from build123d import *

# Parameters (mm, degrees)
SKETCH1_R           = 25
BOSS_EXTRUDE1_DEPTH = 15
CUT_EXTRUDE2_REACH  = 40.406
CUT_EXTRUDE3_DEPTH  = 5


with BuildPart() as part:
    # Sketch1 → Boss-Extrude1 (new body)
    with BuildSketch(Plane(origin=(0, 0, 0), x_dir=(1, 0, 0), z_dir=(0, 1, 0))):
        with Locations(Location((0, 0, 0), (0, 0, 270))):
            Circle(SKETCH1_R)
    extrude(amount=BOSS_EXTRUDE1_DEPTH)

    # Sketch7 → Cut-Extrude2 (cut, up to next)
    with BuildSketch(Plane(origin=(0, 15, 0), x_dir=(1, 0, 0), z_dir=(0, 1, 0)), mode=Mode.PRIVATE) as cut_extrude2_sk1:
        Polygon((0, 5.132643893), (-4.445, 2.566321947), (-4.445, -2.566321947), (0, -5.132643893), (4.445, -2.566321947), (4.445, 2.566321947), align=None)
    cut_extrude2_tool1 = extrude(cut_extrude2_sk1.sketch, amount=-CUT_EXTRUDE2_REACH, mode=Mode.PRIVATE) & part.part
    add(cut_extrude2_tool1.solids().sort_by_distance((0, 15, 0))[0], mode=Mode.SUBTRACT)

    # Sketch8 → Cut-Extrude3 (cut)
    with BuildSketch(Plane.XZ):
        with BuildLine():
            ThreePointArc((2.867832451, 6.276606431), (5.55485913, 5.311303559), (8.103473198, 4.024257195))
            ThreePointArc((8.103473198, 4.024257195), (12.790122891, 3.37163327), (17.445502266, 2.524257195))
            ThreePointArc((17.445502266, 2.524257195), (19.894779582, 1.820498395), (21, -0.475742805))
            ThreePointArc((21, -0.475742805), (19.894779582, -2.771984005), (17.445502266, -3.475742805))
            ThreePointArc((17.445502266, -3.475742805), (12.790122891, -4.32311888), (8.103473198, -4.975742805))
            ThreePointArc((8.103473198, -4.975742805), (5.55485913, -6.262789168), (2.867832451, -7.22809204))
            ThreePointArc((2.867832451, -7.22809204), (0, -7.852228414), (-2.867832451, -7.22809204))
            ThreePointArc((-2.867832451, -7.22809204), (-5.55485913, -6.262789168), (-8.103473198, -4.975742805))
            ThreePointArc((-8.103473198, -4.975742805), (-12.790122891, -4.32311888), (-17.445502266, -3.475742805))
            ThreePointArc((-17.445502266, -3.475742805), (-19.894779582, -2.771984005), (-21, -0.475742805))
            ThreePointArc((-21, -0.475742805), (-19.894779582, 1.820498395), (-17.445502266, 2.524257195))
            ThreePointArc((-17.445502266, 2.524257195), (-12.790122891, 3.37163327), (-8.103473198, 4.024257195))
            ThreePointArc((-8.103473198, 4.024257195), (-5.55485913, 5.311303559), (-2.867832451, 6.276606431))
            ThreePointArc((-2.867832451, 6.276606431), (0, 6.900742805), (2.867832451, 6.276606431))
        make_face()
    extrude(amount=-CUT_EXTRUDE3_DEPTH, mode=Mode.SUBTRACT)


solid = part.part
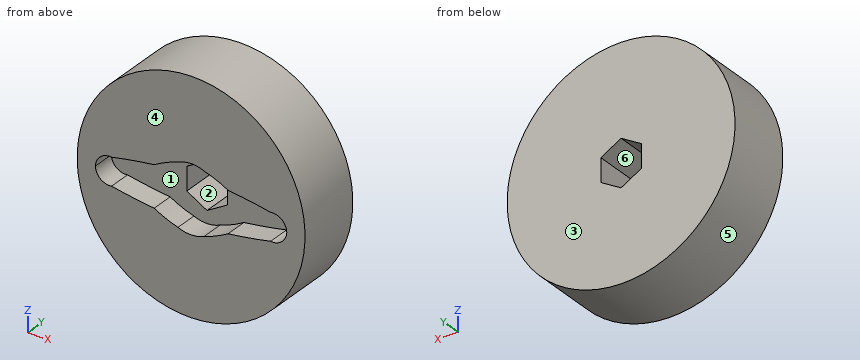
Input: part model. Units: mm. Frame: model coordinates. Face numbers are marked on the shaded views. A direction names the side the tool comes from. Give positions to 0.01 mm unless a question says otherwise; leave off trailing zeros. Loops run counter-clockwise (first coordinate to the right, second up) from the corner with the lowest first, then second, coordinate; pieces in that order, holes last. Notation, with made-up numbers: (14.25, 3) - (52.25, 3) arc R18 ccw to (52.25, 18) - close; hole circle Ø8 at (32, -32.5). An arc over 180 degrees is marked (long way). Use CSV: the item, a comma, the result in double quotes. Start each with the question number.
Item 1: Contact query for flat-ended pins moving along their axis: P1, Ø5, axis at y = 4, z = 5.5, coming from the -X side; P2, Ø1, axis at x = 16, y = 3.5, coming from the +Z side; P3, Ø2.5, axis at y = 8.5, z = 0, coming from the +X side. Output: stop coordinate, or through.
Item 2: Section B-B on z = -6. Return loops of the section in (x, y).
Item 3: Section A-A on y = 2.75. Return loops of the section in (x, z), then the cut area to 3 significant figures.
Item 4: Section D-D on x = -7. Return loops of the section in (y, z), then the cut area to 3 significant figures.
Item 5: Line query: line 1 (X direction, y = 13.5, z = 0) (3 decimals); line 2 (Z direction, x = -3, y = 12); line 3 (Y direction, x = 20, z = 1.5). Output: solid intervals per line, ascending.
Item 6: Mould query, pull axis X, two halves, no side actions, for the marked faces 4, 5 and 6. Classes: pulls with the +X half, pulls with the -X half, needs draft (parallel to the pull), parting line crosses it, or undercut.
Item 7: Reachability of the marked faces 1, 2 and 3 from +Z, -Z, +X, -X, +Y, -Y: full face, straight path, thin tool, end or side. Return the list, or none.
Item 8: Section C-C on y = 7.5. Return loops of the section in (x, z) (3 decimals), then the cut area to 3 significant figures.
Ans:
1,P1,"stops at x = -24.82"
1,P2,"stops at z = 19.62"
1,P3,"stops at x = 25"
2,outline,"(-24.27, 0) - (-6.14, 0) - (-6.14, 5) - (6.14, 5) - (6.14, 0) - (24.27, 0) - (24.27, 15) - (-24.27, 15) - close"
3,outline,"circle Ø50 at (0, 0); hole (-21, -0.48) arc R3.12 ccw to (-17.45, -3.48) arc R113.52 ccw to (-8.1, -4.98) arc R23.27 ccw to (-2.87, -7.23) arc R6.9 ccw to (2.87, -7.23) arc R23.27 ccw to (8.1, -4.98) arc R113.52 ccw to (17.45, -3.48) arc R3.12 ccw to (21, -0.48) arc R3.12 ccw to (17.45, 2.52) arc R113.52 ccw to (8.1, 4.02) arc R23.27 ccw to (2.87, 6.28) arc R6.9 ccw to (-2.87, 6.28) arc R23.27 ccw to (-8.1, 4.02) arc R113.52 ccw to (-17.45, 2.52) arc R3.12 ccw to start"
3,area,"1,580 mm2"
4,outline,"(0, -24) - (15, -24) - (15, 24) - (0, 24) - (0, 4.63) - (5, 4.63) - (5, -5.58) - (0, -5.58) - close"
4,area,"669 mm2"
5,line 1,"x = -25 to -4.445, 4.445 to 25"
5,line 2,"z = -24.82 to -3.4, 3.4 to 24.82"
5,line 3,"y = 5 to 15"
6,face 4,"needs draft"
6,face 5,"parting line crosses it"
6,face 6,"undercut"
7,face 1,"-Y"
7,face 2,"+Y, -Y"
7,face 3,"+Z, -Z, +X, -X, +Y"
8,outline,"circle Ø50 at (0, 0); hole (-4.445, -2.566) - (0, -5.133) - (4.445, -2.566) - (4.445, 2.566) - (0, 5.133) - (-4.445, 2.566) - close"
8,area,"1,900 mm2"
